Here's how the part is built. I have some questions about the finished solid (model axes, mm). Round coordinates to 2 decimals unless told otherwise and drop trailing zeros. Loops run counter-clockwise (first coordinate to the right, second up) from the corner with the lowest first, then second, coordinate; pieces in that order, holes last. Notation, with made-up numbers: M 59,-22.5 L 117,-22.5 A22 ccw 117,12.5 Z; hole C -2.5,-39 d9. An arc over 180 degrees is marked long. Answer as a JSON object with one key per item and string values.
from build123d import *

# Parameters (mm, degrees)
F1_DEPTH = 232


with BuildPart() as f1:
    # F0 (on Front) → F1 (new body)
    with BuildSketch(Plane.XZ):
        with BuildLine():
            Line((22.5, -3), (22.5, 11))
            Line((22.5, 11), (-22.5, 11))
            Line((-22.5, 11), (-22.5, -11))
            Line((-22.5, -11), (-14.187015, -11))
            Line((-14.187015, -11), (-16.271666, -7.018649))
            Line((-16.271666, -7.018649), (-7.329346, -7.018649))
            Line((-7.329346, -7.018649), (-9.875086, -11))
            Line((-9.875086, -11), (14.5, -11))
            ThreePointArc((14.5, -11), (16.843146, -5.343146), (22.5, -3))
        make_face()
    extrude(amount=-F1_DEPTH)


solid = f1.part
Item 1: If I drill on L1, parallel to Z at x = -10, y = 108.5; L2, parallel to X at y = 50, z = -9.5; L3, parallel to Z at x = -8, y = 186, over which ranges is the centre line in solid material (lowest first)? Write a range as from..to.
Solution:
{"L1": "z = -7.02..11", "L2": "x = -22.5..-14.97, -8.92..14.64", "L3": "z = -11..-8.07, -7.02..11"}
Item 2: I want a section at A-A on y = 24.5. List the corners of the cut face in (x, z) for me, plus the area to 3 significant figures.
Solution:
{"outline": "M -22.5,-11 L -14.19,-11 L -16.27,-7.02 L -7.33,-7.02 L -9.88,-11 L 14.5,-11 A8 cw 22.5,-3 L 22.5,11 L -22.5,11 Z", "area": "913 mm2"}
Item 3: We'd pull the mould along X, two halves only. Please class faces 1 (the face through (-18, 114, -11)), 2 (the face through (-12, 114, -7.019)), 3 (the face through (16.781, 114.376, -5.406)): +X half, -X half, draft (parallel to the pull), parting line (faces both ways), or undercut.
Solution:
{"face 1": "draft", "face 2": "undercut", "face 3": "+X half"}
